Source: CAD feature listing. Evaluate the final solid. Frame: model axes, mm. Face numbers are marked on the shaded views. A direction names the side the tool comes from. Round coordinates to 2 decimals unless told otherwise and drop trailing zeros. Order: outer loops, then holes, each group sorted by start corner. A loop starts at its lowest first (then second) coordinate and runs counter-clockwise, first axis right, second up. Notation, with made-up numbers: M -37,-32.5 L 12,-32.5 A25 ccw 12,-11.5 Z; hole C -39.5,-39 d3. An arc over 180 degrees is marked long. Use CSV: the item, a comma, the result in double quotes. Start each with the question number.
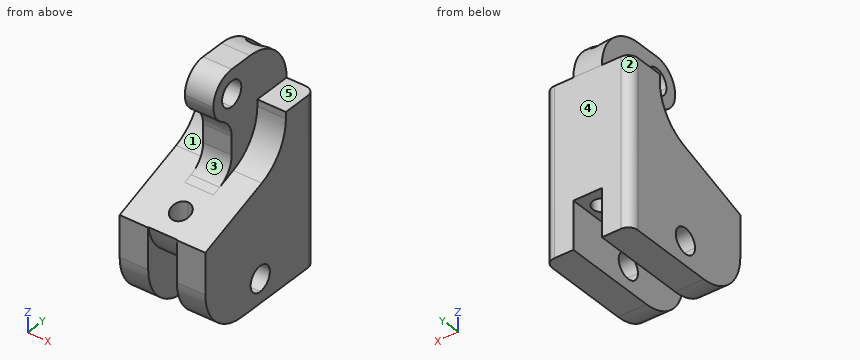
```python
from build123d import *

# Parameters (mm, degrees)
F1_DEPTH     = 15
F3_DEPTH     = 6
F5_DEPTH     = 18
F6_R         = 10
F7_R         = 10
F10_DEPTH    = 6
F11_DEPTH    = 6
F12_R        = 2
F14_DEPTH    = 6
F18_DEPTH    = 40
F20_DEPTH    = 40
F22_DEPTH    = 6
F23_T1_DEPTH = 6


# Not quite as in the source:
# - a fillet or chamfer that OpenCascade refuses, or shapes differently, is made with other operations: its cross-section is extruded or revolved along the edge and cut away or added


with BuildPart() as f1:
    # F0 (on Front) → F1 (new body, symmetric)
    with BuildSketch(Plane.XZ):
        Polygon((9, -12.5), (9, 12.5), (3, 12.5), (3, 22.5), (-3, 22.5), (-3, 12.5), (-9, 12.5), (-9, -12.5), (-9, -22.5), (-3, -22.5), (-3, -12.5), (3, -12.5), (3, -22.5), (9, -22.5), align=None)
    extrude(amount=F1_DEPTH, both=True)

    # F2 (on face) → F3 (cut)
    with BuildSketch(Plane(origin=(-3, 0, 0), x_dir=(0, -1, 0), z_dir=(-1, 0, 0))):
        with BuildLine():
            ThreePointArc((0, 20.12), (-2.62, 17.5), (0, 14.88))
            Line((0, 14.88), (0, 20.12))
        make_face()
        with BuildLine():
            Line((0, 20.12), (0, 14.88))
            ThreePointArc((0, 14.88), (1.8526197667, 15.6473802333), (2.62, 17.5))
            ThreePointArc((2.62, 17.5), (1.8526197667, 19.3526197667), (0, 20.12))
        make_face()
    extrude(amount=-F3_DEPTH, mode=Mode.SUBTRACT)

    # F4 (on face) → F5 (cut)
    with BuildSketch(Plane(origin=(-9, 0, 0), x_dir=(0, -1, 0), z_dir=(-1, 0, 0))):
        with BuildLine():
            ThreePointArc((0, -20.12), (1.8526197667, -19.3526197667), (2.62, -17.5))
            ThreePointArc((2.62, -17.5), (-1.8526197667, -15.6473802333), (0, -20.12))
        make_face()
    extrude(amount=-F5_DEPTH, mode=Mode.SUBTRACT)

    # F6
    f6_edges = [f1.edges().sort_by_distance(p)[0] for p in [
        (0, -15, -12.5),
    ]]
    fillet(f6_edges, radius=F6_R)

    # F7
    f7_edges = [f1.edges().sort_by_distance(p)[0] for p in [
        (0, 15, 22.5),
        (0, -15, 22.5),
        (6, -15, -22.5),
        (-6, -15, -22.5),
    ]]
    fillet(f7_edges, radius=F7_R)

    # F9 (on face) → F10 (cut)
    with BuildSketch(Plane(origin=(-9, 0, 0), x_dir=(0, -1, 0), z_dir=(-1, 0, 0))):
        with BuildLine():
            ThreePointArc((-7, 11.0872004348), (-5.1915204429, 5.3514360713), (-0.4202014333, 1.690274227))
            Line((-0.4202014333, 1.690274227), (15, -3.9222201011))
            Line((15, -3.9222201011), (15, 12.5))
            Line((15, 12.5), (-7, 12.5))
            Line((-7, 12.5), (-7, 11.0872004348))
        make_face()
    extrude(amount=-F10_DEPTH, mode=Mode.SUBTRACT)

    # F8 (on face) → F11 (cut)
    with BuildSketch(Plane.YZ.offset(9)):
        with BuildLine():
            Line((7, 12.5), (-15, 12.5))
            Line((-15, 12.5), (-15, -3.92222))
            Line((-15, -3.92222), (0.4202014333, 1.6902743281))
            ThreePointArc((0.4202014333, 1.6902743281), (5.1915204429, 5.3514361724), (7, 11.087200536))
            Line((7, 11.087200536), (7, 12.5))
        make_face()
    extrude(amount=-F11_DEPTH, mode=Mode.SUBTRACT)

    # F12
    f12_edges = [f1.edges().sort_by_distance(p)[0] for p in [
        (9, 15, -5),
        (-9, 15, -5),
    ]]
    fillet(f12_edges, radius=F12_R)

    # F13 (on face) → F14 (cut)
    with BuildSketch(Plane(origin=(-3, 0, 0), x_dir=(0, -1, 0), z_dir=(-1, 0, 0))):
        with BuildLine():
            Line((5, 22.5), (0, 22.5))
            ThreePointArc((0, 22.5), (3.5355339059, 21.0355339059), (5, 17.5))
            Line((5, 17.5), (5, -0.2825177585))
            Line((5, -0.2825177585), (14.9033390576, -3.8870383953))
            ThreePointArc((14.9033390576, -3.8870383953), (14.9758054957, -3.1952012025), (15, -2.5))
            Line((15, -2.5), (15, 12.5))
            ThreePointArc((15, 12.5), (12.0710678119, 19.5710678119), (5, 22.5))
        make_face()
    extrude(amount=-F14_DEPTH, mode=Mode.SUBTRACT)

    # F17 (on face) → F18 (cut)
    with BuildSketch(Plane.XY.offset(17.5)):
        with BuildLine():
            ThreePointArc((2, -10), (1.4142135624, -8.5857864376), (0, -8))
            Line((0, -8), (0, -12))
            ThreePointArc((0, -12), (1.4142135624, -11.4142135624), (2, -10))
        make_face()
        with BuildLine():
            Line((0, -12), (0, -8))
            ThreePointArc((0, -8), (-2, -10), (0, -12))
        make_face()
    extrude(amount=-F18_DEPTH, mode=Mode.SUBTRACT)

    # F19 (on face) → F20 (cut)
    with BuildSketch(Plane(origin=(0, 0, -12.5), x_dir=(1, 0, 0), z_dir=(0, 0, -1))):
        with BuildLine():
            Line((0, -9), (0, -11))
            Line((0, -11), (0, -13))
            ThreePointArc((0, -13), (1.4142135624, -12.4142135624), (2, -11))
            ThreePointArc((2, -11), (1.4142135624, -9.5857864376), (0, -9))
        make_face()
        with BuildLine():
            Line((0, -13), (0, -11))
            Line((0, -11), (0, -9))
            ThreePointArc((0, -9), (-2, -11), (0, -13))
        make_face()
    extrude(amount=-F20_DEPTH, mode=Mode.SUBTRACT)

    # F21 (on face) → F22 (cut)
    with BuildSketch(Plane.YZ.offset(3)):
        with BuildLine():
            ThreePointArc((0, 12.5), (-3.5355339059, 13.9644660941), (-5, 17.5))
            Line((-5, 17.5), (-5, -0.2825177585))
            Line((-5.0000000325, -0.2825176692), (0, 1.537333514))
            Line((0, 1.537333514), (0, 12.5))
        make_face()
    extrude(amount=-F22_DEPTH, mode=Mode.SUBTRACT)

    # F23: fillet of radius 5 on 2 edges, made by hand

    # F23_s2 → F23_t1 (join)
    with BuildSketch(Plane.YZ.offset(-3)):
        with BuildLine():
            ThreePointArc((-2.5, 13.1698729811), (-0.6698729811, 11.3397459622), (0, 8.8397459622))
            Line((0, 8.8397459622), (0, 12.5))
            ThreePointArc((0, 12.5), (-1.2940952255, 12.6703708686), (-2.5, 13.1698729811))
        make_face()
        with BuildLine():
            ThreePointArc((0, 5.0383711039), (-0.9042397786, 2.1704889222), (-3.2898992834, 0.339908))
            Line((-3.2898992834, 0.339908), (0, 1.537333514))
            Line((0, 1.537333514), (0, 5.0383711039))
        make_face()
    extrude(amount=F23_T1_DEPTH)


solid = f1.part
```
(1) Section C-C on y = -8.5. Return loops of the section in (x, z).
(2) Section D-D on y = 6. Return loops of the section in (x, z).
(3) Reachability of the marked faces 1, 2, 3, 4 and 5 from +Z, -Z, +X, -X, +Y, -Y: full face, straight path, thin tool, end or side. Return the list, or none.
(4) Section A-A on x = 1.25. Return loops of the section in (y, z).
(5) Section B-B on x = -6.5. Return loops of the section in (y, z).
(6) Line query: line 1 along X through (y, z) = (-10, -10.5); line 2 along X through (y, z) = (7.5, -13); line 3 along Z through (x, y) = (3.75, -5). Output: solid intervals per line, ascending.
(7) Contact query for flat-ended pins moving along their axis: P1, Ø16, axis at y = 1.5, z = 14.5, coming from the +X side; P2, Ø1.5, axis at y = 0, z = 11.5, coming from the +X side; P3, Ø0.7, axis at x = 6, z = 12, coming from the -Y side; P4, Ø1.9, axis at x = 0.5, z = 8, coming from the -Y side. Output: stop coordinate, or through.
Results below:
1,outline,"M -9,-21.87 L -3,-21.87 L -3,-11.87 L -1.32,-11.87 L -1.32,-1.56 L -9,-1.56 Z; M 1.32,-11.87 L 3,-11.87 L 3,-21.87 L 9,-21.87 L 9,-1.56 L 1.32,-1.56 Z"
2,outline,"M -9,-22.5 L -3,-22.5 L -3,-12.5 L 3,-12.5 L 3,-22.5 L 9,-22.5 L 9,6.73 L 3,6.73 L 3,22.45 L -3,22.45 L -3,6.73 L -9,6.73 Z"
3,face 1,"+Z, -X, -Y"
3,face 2,"+Z, -Z, -X, +Y"
3,face 3,"+X, -X, -Y"
3,face 4,"+Z, -Z, +X, -X, +Y"
3,face 5,"+Z, +X, +Y, -Y"
4,outline,"M -14.9,-3.89 A10 ccw -11.56,-10.05 L -11.56,-2.67 Z; M -8.44,-11.89 A10 ccw -5,-12.5 L 9.44,-12.5 L 9.44,21.46 A10 ccw 5,22.5 L 0,22.5 A5 ccw -2.5,13.17 A5 cw 0,8.84 L 0,5.04 A5 cw -3.29,0.34 L -8.44,-1.53 Z; M 12.56,-12.5 L 15,-12.5 L 15,12.5 A10 ccw 12.56,19.04 Z; hole C 0,17.5 d5.24"
5,outline,"M -15,-12.5 A10 ccw -5,-22.5 L 15,-22.5 L 15,12.5 L 7,12.5 L 7,11.09 A10 cw 0.42,1.69 L -15,-3.92 Z; hole C 0,-17.5 d5.24"
6,line 1,"x = -9 to -2, 2 to 9"
6,line 2,"x = -9 to -3, 3 to 9"
6,line 3,"z = -22.5 to -0.28"
7,P1,"stops at x = 9"
7,P2,"stops at x = 3"
7,P3,"stops at y = 7"
7,P4,"stops at y = 0"
